For this review, take the finished solid that the model builds, in its own axes (mm). A direction names the side the tool comes from. Coordinates: 2 decimals unless noted, no trailing zeros. Write each loop counter-clockwise with the first axis right and the second up, starting at its lowest first coordinate (ties: lowest second). Pieces come first, ordered by that corner, then holes.
1) We need section D-D on z = 7.5. Write out the cut boundary in (x, y), then the cut area to 3 significant figures.
2) We need section A-A on y = -12.7. Write out the cut boundary in (x, z).
3) We need section C-C on z = 28. Write out the cut boundary in (x, y).
4) Insertion check: P1, Ø2, axis at y = -16.5, z = 11, coming from the +X side; P2, Ø3.5, axis at x = 9, z = 35, coming from the -Y side; P3, Ø12, axis at x = 8.5, z = 38, coming from the +Y side; P4, Ø11.5, axis at x = 25.4, y = -12.7, coming from the +Z side. Each pin has a flat end and moves straight along its axis. Give the tip position at first contact, or say it passes through.
5) For faces 5 (the face through (12.7, -13, 24)), 6 (the face through (6.4, -12.8, 25.4)), list the 3-axis set-ups (+Z, -Z, +X, -X, +Y, -Y) from which the entire face can be reached by the end or side of a thin tool; tool diameter is ignored.
6) Mouldability with a two-part tool opening along Y and no side actions: class faces 1 (the face through (17, -25.4, 9)), 2 (the face through (6, -19.05, 37)), 3 (the face through (34, -13, 12.7)), 4 (the face through (6, -6.35, 37)) as pulls with the +Y half, pulls with the -Y half, needs draft (parallel to the pull), parting line crosses it, or undercut.
7) To check wall thickness, follow line 1 along Y through (x, z) = (25.4, 7.75); line 2 along Z through (x, y) = (52.5, -18.5). State the ranges of each line that lie inside material, in increasing order.
8) We need section B-B on x = 25.4. Write out the cut boundary in (y, z).
from build123d import *

# Parameters (mm, degrees)
F0_W     = 12.7
F0_H     = 31.75
F0_H_2   = 12.7
F0_W_2   = 44.45
F1_DEPTH = 25.4
F2_R     = 6.35
F3_DEPTH = 25.4
F5_DEPTH = 25.4


with BuildPart() as f1:
    # F0 (on Front) → F1 (new body)
    with BuildSketch(Plane.XZ):
        with Locations((6.35, 28.575)):
            Rectangle(F0_W, F0_H)
        with Locations((6.35, 6.35)):
            Rectangle(F0_W, F0_H_2)
        with Locations((34.925, 6.35)):
            Rectangle(F0_W_2, F0_H_2)
    extrude(amount=F1_DEPTH)

    # F2 (on face) → F3 (cut)
    with BuildSketch(Plane.XY.offset(12.7)):
        with Locations((25.4, -12.7)):
            Circle(F2_R)
        with Locations((44.45, -12.7)):
            Circle(F2_R)
        with BuildLine():
            ThreePointArc((44.45, 0), (56.6503530986, -12.7), (44.45, -25.4))
            Line((44.45, -25.4), (57.15, -25.4))
            Line((57.15, -25.4), (57.15, 0))
            Line((57.15, 0), (44.45, 0))
        make_face()
    extrude(amount=-F3_DEPTH, mode=Mode.SUBTRACT)

    # F4 (on face) → F5 (cut)
    with BuildSketch(Plane.YZ.offset(12.7)):
        with BuildLine():
            ThreePointArc((-19.05, 31.75), (-12.7, 25.4), (-6.35, 31.75))
            ThreePointArc((-6.35, 31.75), (-12.7, 38.1), (-19.05, 31.75))
        make_face()
        with BuildLine():
            ThreePointArc((-19.05, 31.75), (-12.7, 38.1), (-6.35, 31.75))
            Line((-6.35, 31.75), (-6.35, 42.7141417))
            ThreePointArc((-6.35, 42.7141417), (-12.7, 44.41561185), (-19.05, 42.7141417))
            Line((-19.05, 42.7141417), (-19.05, 31.75))
        make_face()
        with BuildLine():
            ThreePointArc((-25.4, 31.75), (-23.6899374795, 38.0805050685), (-19.05, 42.7141417))
            Line((-19.05, 42.7141417), (-19.05, 44.45))
            Line((-19.05, 44.45), (-25.4, 44.45))
            Line((-25.4, 44.45), (-25.4, 31.75))
        make_face()
        with BuildLine():
            ThreePointArc((-19.05, 42.7141417), (-12.7, 44.41561185), (-6.35, 42.7141417))
            Line((-6.35, 42.7141417), (-6.35, 44.45))
            Line((-6.35, 44.45), (-19.05, 44.45))
            Line((-19.05, 44.45), (-19.05, 42.7141417))
        make_face()
        with BuildLine():
            Line((-6.35, 44.45), (-6.35, 42.7141417))
            ThreePointArc((-6.35, 42.7141417), (-1.7100625205, 38.0805050685), (0, 31.75))
            Line((0, 31.75), (0, 44.45))
            Line((0, 44.45), (-6.35, 44.45))
        make_face()
    extrude(amount=-F5_DEPTH, mode=Mode.SUBTRACT)


solid = f1.part
Result:
1. outline: (0, -25.4) - (44.45, -25.4) arc R12.71 ccw to (44.45, 0) - (0, 0) - close; hole circle Ø12.7 at (25.4, -12.7); hole circle Ø12.7 at (44.45, -12.7)
1. area: 1,120 mm2
2. outline: (0, 0) - (19.05, 0) - (19.05, 12.7) - (12.7, 12.7) - (12.7, 25.4) - (0, 25.4) - close; (31.75, 0) - (38.1, 0) - (38.1, 12.7) - (31.75, 12.7) - close; (50.8, 0) - (56.65, 0) - (56.65, 12.7) - (50.8, 12.7) - close
3. outline: (0, -25.4) - (12.7, -25.4) - (12.7, -17.82) - (0, -17.82) - close; (0, -7.58) - (12.7, -7.58) - (12.7, 0) - (0, 0) - close
4. P1: stops at x = 56.34
4. P2: stops at y = -25.31
4. P3: stops at y = 0
4. P4: passes through
5. face 5: +Z, +X, +Y, -Y
5. face 6: +Z, +X, -X
6. face 1: pulls with the -Y half
6. face 2: undercut
6. face 3: needs draft
6. face 4: undercut
7. line 1: y = -25.4 to -19.05, -6.35 to 0
7. line 2: z = 0 to 12.7
8. outline: (-25.4, 0) - (-19.05, 0) - (-19.05, 12.7) - (-25.4, 12.7) - close; (-6.35, 0) - (0, 0) - (0, 12.7) - (-6.35, 12.7) - close
